Part model, mm, in its own coordinate system. Face numbers are marked on the shaded views. Round coordinates to 2 decimals unless told otherwise and drop trailing zeros. Write each loop counter-clockwise with the first axis right and the second up, starting at its lowest first coordinate (ties: lowest second). Pieces come first, ordered by that corner, then holes. Notation, with made-up numbers: M -36,16 L -19,16 A22 cw -19,55 Z; hole C -14,-5 d11. An arc over 180 degrees is marked long. Use a Markdown table: item, result. Add a question column.
1) Slice it at D-D on z = 21. Give the number of separate pieces and of enclosed holes in the cut face, plus the area to 3 significant figures.
2) Slice it at C-C on y = 11.5. Write the cut outline in (x, z).
3) Two-plate mould, pull along X, no slides. Class the marked faces 1, 2 and 3: released by +X, released by -X, zero draft, split by the parting line, or undercut.
4) Slice it at A-A on z = 0. Write the cut outline in (x, y).
5) Drop flat-ended pins along their axis: P1, Ø7, axis at x = 26.5, z = -19, coming from the +Y side; P2, Ø5.5, axis at x = -26.5, z = 19, coming from the +Y side; P3, Ø1.5, axis at y = 12, z = -8.5, coming from the -X side. Give the stop position or say it passes through.
6) Wall check: probe 1 along X at (y, z) = (0.95, -19); probe 2 along Z at (x, y) = (-25, 1); probe 3 along Z at (x, y) = (-27, 1). Give the ranges that are in metal, low to high.
7) Slice it at B-B on x = 0. Write the cut outline in (y, z), plus the area to 3 significant figures.
```python
from build123d import *

# Parameters (mm, degrees)
SKETCH1_R           = 3
SKETCH1_R_2         = 22.5
BOSS_EXTRUDE1_DEPTH = 3


with BuildPart() as part:
    # Sketch1 → Boss-Extrude1 (new body)
    with BuildSketch(Plane(origin=(0, 0, 0), x_dir=(1, 0, 0), z_dir=(0, 1, 0))):
        with BuildLine():
            Line((-26.5, 25), (26.5, 25))
            ThreePointArc((26.5, 25), (30.742640687, 23.242640687), (32.5, 19))
            Line((32.5, 19), (32.5, -19))
            ThreePointArc((32.5, -19), (30.742640687, -23.242640687), (26.5, -25))
            Line((26.5, -25), (-26.5, -25))
            ThreePointArc((-26.5, -25), (-30.742640687, -23.242640687), (-32.5, -19))
            Line((-32.5, -19), (-32.5, 19))
            ThreePointArc((-32.5, 19), (-30.742640687, 23.242640687), (-26.5, 25))
        make_face()
        with Locations(Location((-26.5, 19, 0), (0, 0, 270))):
            Circle(SKETCH1_R, mode=Mode.SUBTRACT)
        with Locations(Location((26.5, 19, 0), (0, 0, 270))):
            Circle(SKETCH1_R, mode=Mode.SUBTRACT)
        with Locations(Location((26.5, -19, 0), (0, 0, 270))):
            Circle(SKETCH1_R, mode=Mode.SUBTRACT)
        with Locations(Location((-26.5, -19, 0), (0, 0, 270))):
            Circle(SKETCH1_R, mode=Mode.SUBTRACT)
        with Locations(Location((0, 0, 0), (0, 0, 270))):
            Circle(SKETCH1_R_2, mode=Mode.SUBTRACT)
    extrude(amount=BOSS_EXTRUDE1_DEPTH)

    # Sketch2 → Revolve3 (revolve)
    with BuildSketch(Plane.XY, mode=Mode.PRIVATE) as revolve3_sk:
        with BuildLine():
            Line((-18.643274342, 4.403733341), (-8.616164915, 12.817477163))
            ThreePointArc((-8.616164915, 12.817477163), (-7.85514437, 13.320291088), (-7, 13.637627215))
            Line((-7, 13.637627215), (-6.283760857, 10.724381347))
            ThreePointArc((-6.283760857, 10.724381347), (-6.49754695, 10.645047315), (-6.687802086, 10.519343834))
            Line((-6.687802086, 10.519343834), (-16.714911513, 2.105600012))
            ThreePointArc((-16.714911513, 2.105600012), (-19.42181871, 0.542766413), (-22.5, 0))
            Line((-22.5, 0), (-22.5, 3))
            ThreePointArc((-22.5, 3), (-20.44787914, 3.361844275), (-18.643274342, 4.403733341))
        make_face()
    revolve(revolve3_sk.sketch.rotate(Axis((0, 0, 0), (0, 1, 0)), 180), axis=Axis((0, 0, 0), (0, 1, 0)))


solid = part.part
```
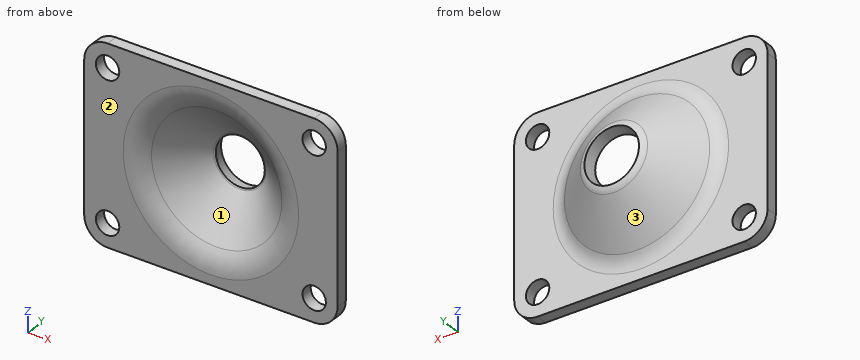
Entries:
| question | item | result |
|---|---|---|
| 1 | separate pieces | 3 |
| 1 | enclosed holes | 0 |
| 1 | area | 167 mm^2 |
| 2 | outline | C 0,0 d20.37; hole C 0,0 d12.95 |
| 3 | face 1 | undercut |
| 3 | face 2 | zero draft |
| 3 | face 3 | split by the parting line |
| 4 | outline | M -32.5,0 L -22.5,0 A9 ccw -16.71,2.11 L -6.69,10.52 A1 cw -6.28,10.72 L -7,13.64 A4 ccw -8.62,12.82 L -18.64,4.4 A6 cw -22.5,3 L -32.5,3 Z; M 6.28,10.72 A1 cw 6.69,10.52 L 16.71,2.11 A9 ccw 22.5,0 L 32.5,0 L 32.5,3 L 22.5,3 A6 cw 18.64,4.4 L 8.62,12.82 A4 ccw 7,13.64 Z |
| 5 | P1 | stops at y = 3 |
| 5 | P2 | passes through |
| 5 | P3 | stops at x = -6.44 |
| 6 | probe 1 | x = -32.5 to -29.5, -23.5 to 23.5, 29.5 to 32.5 |
| 6 | probe 2 | z = -25 to -21.6, -16.4 to 16.4, 21.6 to 25 |
| 6 | probe 3 | z = -24.98 to -21.96, -16.04 to 16.04, 21.96 to 24.98 |
| 7 | outline | M 0,-25 L 3,-25 L 3,-22.5 A6 cw 4.4,-18.64 L 12.82,-8.62 A4 ccw 13.64,-7 L 10.72,-6.28 A1 cw 10.52,-6.69 L 2.11,-16.71 A9 ccw 0,-22.5 Z; M 0,22.5 A9 ccw 2.11,16.71 L 10.52,6.69 A1 cw 10.72,6.28 L 13.64,7 A4 ccw 12.82,8.62 L 4.4,18.64 A6 cw 3,22.5 L 3,25 L 0,25 Z |
| 7 | area | 132 mm^2 |
